Input: part model. Units: mm. Frame: model coordinates. A direction names the side the tool comes from. Give positions to 0.01 mm unless a question says otherwise; leave off trailing zeros. Write each loop counter-clockwise with the first axis right and the second up, starting at its lowest first coordinate (ties: lowest second). Pieces come first, ordered by that corner, then holes. Notation, with made-up numbers: (66.25, 36.25) - (85.25, 36.25) arc R9 ccw to (85.25, 41.25) - close; hole circle Ø7 at (32.25, 22.5). An arc over 180 degrees is marked (long way). Use a Markdown table: item, result. Add a question column.
1. Section query A-A, the plane x = 38.5. Return loops of the section in (y, z), plus the area to 3 significant figures.
2. Mould query, pull axis Z, two halves, no side actions, for faces 4 (the flat face through (0.585, -1.007, 6.162)), 5 (the cylindrical face through (13.8, -1, 35.9)), 6 (the flat face through (-1, 9, 12.5)), 7 (the cylindrical face through (55.69, -0.99, 36.33)). Classes: released by +Z, released by -Z, zero draft, split by the parting line, or undercut.
3. Section query C-C, the plane z = 20. Return loops of the section in (x, y), plus the area to 3 significant figures.
4. Pin query (flat end, axial travel): pin 1 (20 mm diameter, centred on x = 17.5, z = 23.5, fed in from +Y); pin 2 (0.8 mm diameter, centred on x = -0.5, y = 5.5, fed in from +Z); pin 3 (4.5 mm diameter, centred on y = 13.5, z = 23.5, fed in from +X). Return the tip coordinate at first contact, or that it passes through.
5. Set-up query: faces 1 (the flat face through (0.585, -1.007, 33.662)), 2 (the flat face through (0, 11, 20)), 3 (the cylindrical face through (56.43, -0.99, 4.55)). Return all of +Z, -Z, +X, -X, +Y, -Y with unobstructed straight access to the full face (end or side cutting, diameter ignored); none if empty.
6. Material intervals for probe 1 along X at (y, z) = (-1.2, 35); probe 2 along Y at (x, z) = (41, 34.5), sorted ascending.
7. Section query B-B, the plane y = 13. Return loops of the section in (x, z).
8. Section query D-D, the plane x = 15. Return loops of the section in (y, z), plus the area to 3 significant figures.
```python
from build123d import *

# Parameters (mm, degrees)
SM_BASE_FLANGE_1_DEPTH       = 40
CUT_EXTRUDE_1_REACH          = 77.392
SKETCH_6_R                   = 12.5
HOLE_WIZARD_M3_2_D           = 3
HOLE_WIZARD_M3_4_D           = 3
HOLE_WIZARD_M3_1_D           = 3.4
HOLE_WIZARD_M3_1_CSINK_D     = 6.3
HOLE_WIZARD_M3_1_CSINK_ANGLE = 90
CUT_EXTRUDE_2_DEPTH          = 12.5
CUT_EXTRUDE_START            = 27.5
CUT_EXTRUDE_2_2_DEPTH        = 12.5


# Read off the part's stored shape, not the designer's step: 除料-伸長2
# Sheet-metal steps are written as plain solids
with BuildPart() as part:
    # Sketch 1 → 基材-凸緣1 (new body)
    with BuildSketch(Plane.XY):
        with BuildLine():
            Line((0, 20), (0, 0.7366))
            ThreePointArc((0, 0.7366), (0.215745145, 0.215745145), (0.7366, 0))
            Line((0.7366, 0), (60, 0))
            Line((60, 0), (60, -2))
            Line((60, -2), (0.7366, -2))
            ThreePointArc((0.7366, -2), (-1.198468417, -1.198468417), (-2, 0.7366))
            Line((-2, 0.7366), (-2, 20))
            Line((-2, 20), (0, 20))
        make_face()
    extrude(amount=SM_BASE_FLANGE_1_DEPTH)

    # 草圖6 → 除料-伸長1 (cut, up to next)
    with BuildSketch(Plane(origin=(0, -2, 0), x_dir=(-1, 0, 0), z_dir=(0, -1, 0)), mode=Mode.PRIVATE) as cut_extrude_1_sk1:
        with Locations(Location((-35, -20, 0), (0, 0, 90))):
            Circle(SKETCH_6_R)
    cut_extrude_1_tool1 = extrude(cut_extrude_1_sk1.sketch, amount=-CUT_EXTRUDE_1_REACH, mode=Mode.PRIVATE) & part.part
    add(cut_extrude_1_tool1.solids().sort_by_distance((35, -2, 20))[0], mode=Mode.SUBTRACT)

    # M3 螺紋孔2 (through all)
    with Locations(Plane.ZY.offset(2)):
        with Locations((20, 13)):
            Hole(HOLE_WIZARD_M3_2_D / 2)

    # M3 螺紋孔4 (through all)
    with Locations(Plane(origin=(0, -2, 0), x_dir=(-1, 0, 0), z_dir=(0, -1, 0))):
        with Locations((-15, -5), (-55, -5), (-55, -35), (-15, -35)):
            Hole(HOLE_WIZARD_M3_4_D / 2)

    # M3 平錐坑頭螺釘的錐孔1 (through all)
    with Locations(Plane(origin=(0, -2, 0), x_dir=(-1, 0, 0), z_dir=(0, -1, 0))):
        with Locations((-46.313708499, -8.686291501), (-46.313708499, -31.313708499), (-23.686291501, -31.313708499), (-23.686291501, -8.686291501)):
            CounterSinkHole(HOLE_WIZARD_M3_1_D / 2, HOLE_WIZARD_M3_1_CSINK_D / 2, counter_sink_angle=HOLE_WIZARD_M3_1_CSINK_ANGLE)

    # 除料-伸長2 outline → 除料-伸長2 (cut)
    with BuildSketch(Plane.XY):
        with BuildLine():
            Line((0.5, -1.989752875), (0.672915296, 0.002758179))
            ThreePointArc((0.672915296, 0.002758179), (0.193695905, 0.238770005), (0, 0.7366))
            Line((0, 0.7366), (0, 20))
            Line((0, 20), (-2, 20))
            Line((-2, 20), (-2, 0.7366))
            ThreePointArc((-2, 0.7366), (-1.280385265, -1.112926966), (0.5, -1.989752875))
        make_face()
    extrude(amount=CUT_EXTRUDE_2_DEPTH, mode=Mode.SUBTRACT)

    # Cut-Extrude 2 2 outline → Cut-Extrude 2 2 (cut)
    with BuildSketch(Plane.XY.offset(CUT_EXTRUDE_START)):
        with BuildLine():
            Line((0.5, -1.989752875), (0.672915296, 0.002758179))
            ThreePointArc((0.672915296, 0.002758179), (0.193695905, 0.238770005), (0, 0.7366))
            Line((0, 0.7366), (0, 20))
            Line((0, 20), (-2, 20))
            Line((-2, 20), (-2, 0.7366))
            ThreePointArc((-2, 0.7366), (-1.280385265, -1.112926966), (0.5, -1.989752875))
        make_face()
    extrude(amount=CUT_EXTRUDE_2_2_DEPTH, mode=Mode.SUBTRACT)


solid = part.part
```
Result sheet:
| question | item | result |
|---|---|---|
| 1 | outline | (-2, 0) - (0, 0) - (0, 8) - (-2, 8) - close; (-2, 32) - (0, 32) - (0, 40) - (-2, 40) - close |
| 1 | area | 32.0 mm² |
| 2 | face 4 | zero draft |
| 2 | face 5 | undercut |
| 2 | face 6 | released by -Z |
| 2 | face 7 | undercut |
| 3 | outline | (-2, 0.74) arc R2.74 ccw to (0.74, -2) - (22.5, -2) - (22.5, 0) - (0.74, 0) arc R0.74 cw to (0, 0.74) - (0, 11.5) - (-2, 11.5) - close; (-2, 14.5) - (0, 14.5) - (0, 20) - (-2, 20) - close; (47.5, -2) - (60, -2) - (60, 0) - (47.5, 0) - close |
| 3 | area | 107 mm² |
| 4 | pin 1 | stops at y = 0 |
| 4 | pin 2 | stops at z = 27.5 |
| 4 | pin 3 | stops at x = 0 |
| 5 | face 1 | +Z, -X, +Y |
| 5 | face 2 | +Z, -Z, +X, +Y |
| 5 | face 3 | +Y, -Y |
| 6 | probe 1 | x = 0.57 to 13.5, 16.5 to 53.5, 56.5 to 60 |
| 6 | probe 2 | y = -2 to 0 |
| 7 | outline | (-2, 12.5) - (0, 12.5) - (0, 18.5) - (-2, 18.5) - close; (-2, 21.5) - (0, 21.5) - (0, 27.5) - (-2, 27.5) - close |
| 8 | outline | (-2, 0) - (0, 0) - (0, 3.5) - (-2, 3.5) - close; (-2, 6.5) - (0, 6.5) - (0, 33.5) - (-2, 33.5) - close; (-2, 36.5) - (0, 36.5) - (0, 40) - (-2, 40) - close |
| 8 | area | 68.0 mm² |
